```python
from build123d import *

# Parameters (mm, degrees)
SKETCH_1_R          = 10.3
EXTRUDE_1_DEPTH     = 2.4
SKETCH_2_R          = 4.3
SKETCH_2_R_2        = 2.9
EXTRUDE_2_DEPTH     = 3.1
SKETCH_3_R          = 0.775
CUT_EXTRUDE_1_DEPTH = 2.4
CUT_EXTRUDE_2_REACH = 7.5
SKETCH_4_R          = 1.4


with BuildPart() as part:
    # 草图1 → 凸台-拉伸1 (new body)
    with BuildSketch(Plane(origin=(0, 0, 0), x_dir=(1, 0, 0), z_dir=(0, 1, 0))):
        Circle(SKETCH_1_R)
    extrude(amount=EXTRUDE_1_DEPTH)

    # 草图2 → 凸台-拉伸2 (add)
    with BuildSketch(Plane(origin=(0, 2.4, 0), x_dir=(1, 0, 0), z_dir=(0, 1, 0))):
        Circle(SKETCH_2_R)
        Circle(SKETCH_2_R_2, mode=Mode.SUBTRACT)
    extrude(amount=EXTRUDE_2_DEPTH)

    # 草图3 → 切除-拉伸1 (cut)
    with BuildSketch(Plane.XZ):
        with Locations((0, 7.1)):
            Circle(SKETCH_3_R)
        with BuildLine():
            ThreePointArc((3.009055484, 6.430830825), (3.066525057, 6.403625854), (3.123748696, 6.375907315))
            ThreePointArc((3.123748696, 6.375907315), (3.734726327, 7.798987329), (3.009055484, 6.430830825))
        make_face()
        with BuildLine():
            ThreePointArc((-6.430830825, 3.009055484), (-6.403625854, 3.066525057), (-6.375907315, 3.123748696))
            ThreePointArc((-6.375907315, 3.123748696), (-7.798987329, 3.734726327), (-6.430830825, 3.009055484))
        make_face()
        with Locations((7.1, 3.4)):
            Circle(SKETCH_3_R)
        with Locations((-7.1, 0)):
            Circle(SKETCH_3_R)
        with Locations((7.1, 0)):
            Circle(SKETCH_3_R)
        with Locations((0, -7.1)):
            Circle(SKETCH_3_R)
        with Locations((3.4, -7.1)):
            Circle(SKETCH_3_R)
    cut_extrude_1 = extrude(amount=-CUT_EXTRUDE_1_DEPTH, mode=Mode.SUBTRACT)

    # 镜向1: 切除-拉伸1 across plane
    add(cut_extrude_1.mirror(Plane(origin=(0, 0, 0), x_dir=(0, 0, 1), z_dir=(1, 0, 0))), mode=Mode.SUBTRACT)

    # 镜向2: 切除-拉伸1 across plane
    add(cut_extrude_1.mirror(Plane.XY), mode=Mode.SUBTRACT)

    # 草图4 → 切除-拉伸2 (cut, up to next)
    with BuildSketch(Plane.XZ, mode=Mode.PRIVATE) as cut_extrude_2_sk1:
        Circle(SKETCH_4_R)
    cut_extrude_2_tool1 = extrude(cut_extrude_2_sk1.sketch, amount=-CUT_EXTRUDE_2_REACH, mode=Mode.PRIVATE) & part.part
    add(cut_extrude_2_tool1.solids().sort_by_distance((0, 0, 0))[0], mode=Mode.SUBTRACT)


solid = part.part
```
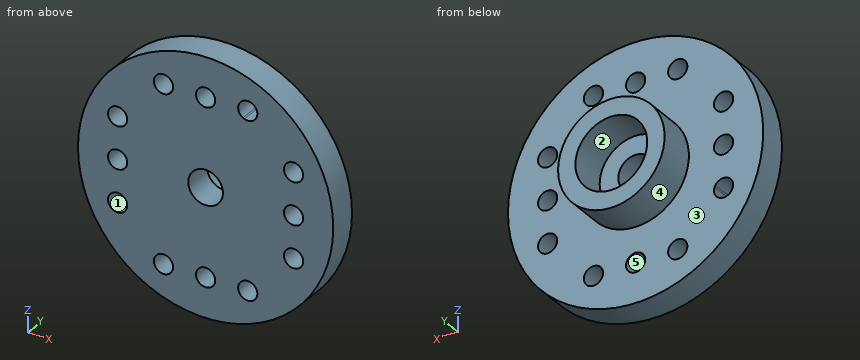
For this review, take the finished solid that the model builds, in its own axes (mm). Face numbers are marked on the shaded views. A direction names the side the tool comes from. Round coordinates to 2 decimals unless told otherwise and drop trailing zeros. Write each loop counter-clockwise with the first axis right and the second up, starting at its lowest first coordinate (ties: lowest second). Pieces come first, ordered by that corner, then holes. Notation, with made-up numbers: (85, 5) -> (132, 5) arc R31 cw to (132, 33) -> close; hole circle Ø11 at (28, 55). An arc over 180 degrees is marked (long way). One line per question, with ' | ' between items. Start each with the question number.
1) For pin 1 Ø3 at (x, z) = (0, 0) entering from +Y; pin 2 Ø3 at (x, y) = (-2, 1) entering from +Z; pin 3 Ø1 at (x, y) = (-5.5, 1) entering from -Z (3 decimals), all flat-tipped, find the tip position at first contact; note any pin that passes through.
2) Add section B-B (y = 2.15). Count the separate pieces of the cut face and the enclosed holes in it, and give its area (3 significant figures).
3) Wall thickness on line 1 along Z through (x, y) = (3.75, 0.95); line 2 along Z through (x, y) = (-7.1, 1.85) (3 decimals); line 3 along X through (y, z) = (1.15, -2.75): over which ranges is each line inside the solid? List them lowest first.
4) Add section A-A (x = 0). Write out the cut boundary in (y, z) (3 decimals), and give its area (3 significant figures).
5) Machinability: for the marked faces 1 and 2, which of the approach directions +Z, -Z, +X, -X, +Y, -Y give a long, thin tool a straight path to every point of the face, cutting with its end or side? Answer none if there is none.
6) Add section D-D (z = 7.1). Write out the cut boundary in (x, y) (3 decimals), and give its area (3 significant figures).
7) Add section C-C (z = -3.75). Write out the cut boundary in (x, y).
8) Mouldability with a two-part tool opening along Z and no side actions: class the marked faces 3, 4 and 5 as +Z half, -Z half, draft (parallel to the pull), parting line (faces both ways), or undercut.
Reported:
1) pin 1: stops at y = 2.4 | pin 2: stops at z = 10.29 | pin 3: stops at z = -9.005
2) separate pieces: 1 | enclosed holes: 13 | area: 304 mm²
3) line 1: z = -9.59 to -7.79, -6.41 to 6.41, 7.79 to 9.59 | line 2: z = -7.462 to -4.175, -2.625 to -0.775, 0.775 to 2.625, 4.175 to 7.462 | line 3: x = -9.93 to -7.52, -6.68 to 6.68, 7.52 to 9.93
4) outline: (0, -10.3) -> (2.4, -10.3) -> (2.4, -7.875) -> (0, -7.875) -> close; (0, -6.325) -> (2.4, -6.325) -> (2.4, -4.3) -> (5.5, -4.3) -> (5.5, -2.9) -> (2.4, -2.9) -> (2.4, -1.4) -> (0, -1.4) -> close; (0, 1.4) -> (2.4, 1.4) -> (2.4, 2.9) -> (5.5, 2.9) -> (5.5, 4.3) -> (2.4, 4.3) -> (2.4, 6.325) -> (0, 6.325) -> close; (0, 7.875) -> (2.4, 7.875) -> (2.4, 10.3) -> (0, 10.3) -> close | area: 44.0 mm²
5) face 1: +Y, -Y | face 2: +Y
6) outline: (-7.462, 0) -> (-4.175, 0) -> (-4.175, 2.4) -> (-7.462, 2.4) -> close; (-2.625, 0) -> (-0.775, 0) -> (-0.775, 2.4) -> (-2.625, 2.4) -> close; (0.775, 0) -> (2.625, 0) -> (2.625, 2.4) -> (0.775, 2.4) -> close; (4.175, 0) -> (7.462, 0) -> (7.462, 2.4) -> (4.175, 2.4) -> close | area: 24.7 mm²
7) outline: (-9.59, 0) -> (-7.79, 0) -> (-7.79, 2.4) -> (-9.59, 2.4) -> close; (-6.41, 0) -> (6.41, 0) -> (6.41, 2.4) -> (2.1, 2.4) -> (2.1, 5.5) -> (-2.1, 5.5) -> (-2.1, 2.4) -> (-6.41, 2.4) -> close; (7.79, 0) -> (9.59, 0) -> (9.59, 2.4) -> (7.79, 2.4) -> close
8) face 3: draft | face 4: parting line | face 5: undercut
